Source: CAD feature listing. Evaluate the final solid. Frame: model axes, mm. A direction names the side the tool comes from. Give positions to 0.01 mm unless a question says otherwise; leave off trailing zeros. Write each loop counter-clockwise with the first axis right and the second up, starting at its lowest first coordinate (ties: lowest second). Pieces come first, ordered by that corner, then holes. Notation, with made-up numbers: (-35.75, -19.75) -> (14.25, -19.75) arc R22 ccw to (14.25, 13.25) -> close; hole circle Ø6 at (0.5, 3.5). An arc over 180 degrees is marked (long way). Write item = value, one per line.
from build123d import *

# Parameters (mm, degrees)
F1_DEPTH = 609.6
F2_W     = 533.4
F2_H     = 127
F2_H_2   = 152.4
F3_DEPTH = 596.9


# Not quite as in the source:
# - a feature names something its author has since deleted; it is built from what else it names


with BuildPart() as f1:
    # F0 (on Right) → F1 (new body)
    with BuildSketch(Plane.YZ):
        Polygon((-584.2, 0), (0, 0), (0, 825.5), (-660.4, 825.5), (-660.4, 101.6), (-584.2, 101.6), align=None)
    extrude(amount=F1_DEPTH)

    # F2 (on face) → F3 (cut)
    with BuildSketch(Plane.XZ.offset(660.4)):
        with Locations((304.8, 723.9)):
            Rectangle(F2_W, F2_H)
        with Locations((304.8, 558.8)):
            Rectangle(F2_W, F2_H)
        with Locations((304.8, 393.7)):
            Rectangle(F2_W, F2_H)
        with Locations((304.8, 215.9)):
            Rectangle(F2_W, F2_H_2)
    extrude(amount=-F3_DEPTH, mode=Mode.SUBTRACT)


solid = f1.part
1) Draft query along X for faces 4 (the flat face through (301, 0, 407)), 5 (the flat face through (571.5, -366, 723)), 6 (the flat face through (0, -335, 419)). Return one class per face: pulls with the +X half, pulls with the -X half, needs draft (parallel to the pull), parting line crosses it, or undercut.
Computed:
face_4 = needs draft
face_5 = undercut
face_6 = pulls with the -X half
2) Access query for faces 1 (the flat face through (301, -623, 101.6)), 2 (the flat face through (301, -296, 0)), 3 (the flat face through (301, -366, 292.1)). Directions: +Z, -Z, +X, -X, +Y, -Y. A direction counts if a zero-diameter tool reaches every point of the face in a straight line with its end or side. Return the directions, or none.
Computed:
face_1 = -Z, +X, -X, -Y
face_2 = -Z, +X, -X, +Y, -Y
face_3 = -Y
3) Contact query for a flat-ended pin moving along its axis: pin 1 (8 mm diameter, centred on x = 428, z = 584.5, fed in from -Y). Output: stop coordinate, or through.
Computed:
pin_1 = -63.5
4) Cut plane B-B (x = 152). Return the cut outline in (y, z), then the cut area to 3 significant figures.
Computed:
outline = (-660.4, 101.6) -> (-584.2, 101.6) -> (-584.2, 0) -> (0, 0) -> (0, 825.5) -> (-660.4, 825.5) -> (-660.4, 787.4) -> (-63.5, 787.4) -> (-63.5, 660.4) -> (-660.4, 660.4) -> (-660.4, 622.3) -> (-63.5, 622.3) -> (-63.5, 495.3) -> (-660.4, 495.3) -> (-660.4, 457.2) -> (-63.5, 457.2) -> (-63.5, 330.2) -> (-660.4, 330.2) -> (-660.4, 292.1) -> (-63.5, 292.1) -> (-63.5, 139.7) -> (-660.4, 139.7) -> close
area = 219,000 mm²
5) Material intervals for L1, parallel to Z at x = 269, y = -249; L2, parallel to X at y = -614, z = 234; L3, parallel to Y at x = 332.5, z = 283, sorted ascending.
Computed:
L1 = 0 to 139.7, 292.1 to 330.2, 457.2 to 495.3, 622.3 to 660.4, 787.4 to 825.5
L2 = 0 to 38.1, 571.5 to 609.6
L3 = -63.5 to 0
6) Cut plane C-C (z = 275). Return the cut outline in (x, y), then the cut area to 3 significant figures.
Computed:
outline = (0, -660.4) -> (38.1, -660.4) -> (38.1, -63.5) -> (571.5, -63.5) -> (571.5, -660.4) -> (609.6, -660.4) -> (609.6, 0) -> (0, 0) -> close
area = 84,200 mm²
7) Cut plane A-A (y = -397). Return the cut outline in (x, z), then the cut area to 3 significant figures.
Computed:
outline = (0, 0) -> (609.6, 0) -> (609.6, 825.5) -> (0, 825.5) -> close; hole (38.1, 139.7) -> (571.5, 139.7) -> (571.5, 292.1) -> (38.1, 292.1) -> close; hole (38.1, 330.2) -> (571.5, 330.2) -> (571.5, 457.2) -> (38.1, 457.2) -> close; hole (38.1, 495.3) -> (571.5, 495.3) -> (571.5, 622.3) -> (38.1, 622.3) -> close; hole (38.1, 660.4) -> (571.5, 660.4) -> (571.5, 787.4) -> (38.1, 787.4) -> close
area = 219,000 mm²
